from build123d import *

# Parameters (mm, degrees)
CHAMFER1_SIZE     = 0.254
CIRPATTERN1_COUNT = 6


with BuildPart() as part:
    # Sketch1 → Revolve1 (revolve)
    with BuildSketch(Plane(origin=(0, 0, 0), x_dir=(0, 0, -1), z_dir=(1, 0, 0)), mode=Mode.PRIVATE) as revolve1_sk:
        Polygon((0, 16.7005), (0, 10.795), (-0.973909372, 10.795), (-0.6604, 9.017), (-1.1684, 9.017), (-1.1684, 6.35), (-7.62, 6.35), (-7.62, 16.7005), align=None)
    revolve(revolve1_sk.sketch.rotate(Axis((0, 0, 0), (0, 0, 1)), 90), axis=Axis((0, 0, 0), (0, 0, 1)))

    # Chamfer1
    chamfer1_edges = [part.edges().sort_by_distance(p)[0] for p in [
        (16.7005, 0, 0),
        (16.7005, 0, 7.62),
    ]]
    chamfer(chamfer1_edges, length=CHAMFER1_SIZE)

    # Sketch2 → 11/64 (0.17188) Diameter Hole2 (revolve, cut)
    with BuildSketch(Plane.YZ.offset(13.4874)):
        Polygon((0, 0), (0, 7.62), (2.3114, 7.62), (2.182876, 7.491476), (2.182876, 0.128524), (2.3114, 0), align=None)
    f_11_64_0_17188_diameter_hole2 = revolve(axis=Axis((13.4874, 0, -6.35), (0, 0, 1)), mode=Mode.SUBTRACT)

    # CirPattern1: 11/64 (0.17188) Diameter Hole2 ×6 about axis
    cirpattern1_axis = Axis((0, 0, 0), (0, 0, 1))
    for i in range(1, CIRPATTERN1_COUNT):
        add(f_11_64_0_17188_diameter_hole2.rotate(cirpattern1_axis, i * 360 / CIRPATTERN1_COUNT), mode=Mode.SUBTRACT)


solid = part.part
Build history of the part. All positions in model axes, mm. Give positions to 0.01 mm unless a question says otherwise; leave off trailing zeros. Order: outer loops, then holes, each group sorted by start corner. A loop starts at its lowest first (then second) coordinate and runs counter-clockwise, first axis right, second up. Notation, with made-up numbers: M -22,63.25 L 24,63.25 A15 ccw 24,77.25 Z; hole C -37,38.25 d6. An arc over 180 degrees is marked long. Put each result on its own line as item: value.
Item 1: Wall check: probe 1 along Y at (x, z) = (0, 6); probe 2 along Y at (x, z) = (-7.5, 5.5); probe 3 along Y at (x, z) = (-5, 3). Give the ranges that are in metal, low to high.
Results are:
probe 1: -16.7 to -6.35, 6.35 to 16.7
probe 2: -14.92 to -13.73, -9.63 to 9.63, 13.73 to 14.92
probe 3: -15.93 to -12.99, -10.37 to -3.91, 3.91 to 10.37, 12.99 to 15.93
Item 2: Cut at C-C on y = 0. Count the separate pieces of the cut face and the enclosed holes in it, then the cut area to 3 significant figures.
Results are:
separate pieces: 4
enclosed holes: 0
area: 81.9 mm2
Item 3: Drop flat-ended pins along their axis: pin 1 Ø3.5 at (x, y) = (-6.74, -11.68) entering from +Z; pin 2 Ø1.5 at (x, z) = (-8, 1.5) entering from -Y; pin 3 Ø6 at (x, y) = (-13, 10.5) entering from -Z; pin 4 Ø1 at (y, z) = (-11, 4.5) entering from -X. Give the stop position or say it passes through.
Results are:
pin 1: through
pin 2: y = -15.04
pin 3: z = 0
pin 4: x = -12.99
Item 4: Pull direction X, two halves, no side cores. Call faces 1 (the face through (-5.415, 9.948, 3.758)), 2 (the face through (-15.93, -5.02, 3.76)), 3 (the face through (7, 0, 7.62)): +X half, -X half, draft (parallel to the pull), parting line (faces both ways), or undercut.
Results are:
face 1: undercut
face 2: parting line
face 3: draft
Item 5: Cut at B-B on z = 6.5. Write the cut outline in (x, y).
Results are:
outline: C 0,0 d33.4; hole C -13.49,0 d4.37; hole C -6.74,-11.68 d4.37; hole C -6.74,11.68 d4.37; hole C 0,0 d12.7; hole C 6.74,-11.68 d4.37; hole C 6.74,11.68 d4.37; hole C 13.49,0 d4.37
